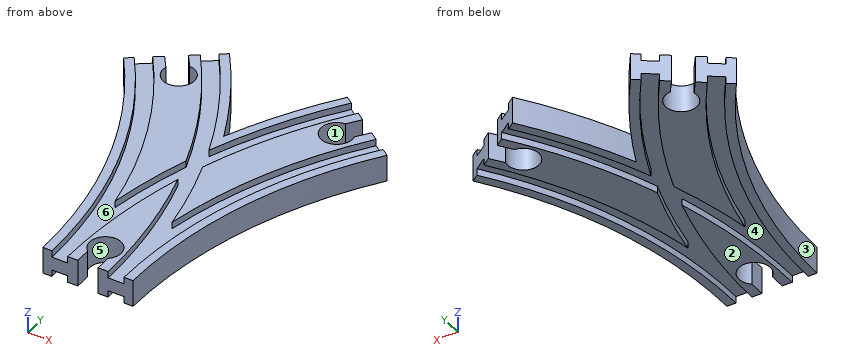
```python
from build123d import *

# Parameters (mm, degrees)
SKETCH003_W          = 7
SKETCH003_H          = 3
SKETCH004_W          = 7
SKETCH004_H          = 3
SKETCH005_W          = 7
SKETCH005_H          = 3
SKETCH006_W          = 7
SKETCH006_H          = 3
POCKET_DEPTH         = 6.001
POCKET_DEPTH_BACK    = -6.001
POCKET001_DEPTH      = 6.001
POCKET001_DEPTH_BACK = -6.001
POCKET002_DEPTH      = 6.001
POCKET002_DEPTH_BACK = -6.001


with BuildPart() as part:
    # AdditivePipe: sweep along a path in Sketch
    with BuildLine(Plane.XY) as additivepipe_path:
        ThreePointArc((0, 0), (-10.865453, 68.601773), (-42.398227, 130.488326))
    # Sketch002 → AdditivePipe (sweep)
    with BuildSketch(Plane.XZ):
        Polygon((-20, 6), (-20, -6), (-16, -6), (-16, -3), (-9, -3), (-9, -6), (9, -6), (9, -3), (16, -3), (16, -6), (20, -6), (20, 6), (16, 6), (16, 3), (9, 3), (9, 6), (-9, 6), (-9, 3), (-16, 3), (-16, 6), align=None)
    sweep(path=additivepipe_path.line)

    # AdditivePipe001: sweep along a path in Sketch001
    with BuildLine(Plane.XY) as additivepipe001_path:
        ThreePointArc((42.398227, 130.488326), (10.865453, 68.601773), (0, 0))
    # Sketch002 → AdditivePipe001 (sweep)
    with BuildSketch(Plane.XZ):
        Polygon((-20, 6), (-20, -6), (-16, -6), (-16, -3), (-9, -3), (-9, -6), (9, -6), (9, -3), (16, -3), (16, -6), (20, -6), (20, 6), (16, 6), (16, 3), (9, 3), (9, 6), (-9, 6), (-9, 3), (-16, 3), (-16, 6), align=None)
    sweep(path=additivepipe001_path.line)

    # SubtractivePipe: sweep along a path in Sketch
    with BuildLine(Plane.XY) as subtractivepipe_path:
        ThreePointArc((0, 0), (-10.865453, 68.601773), (-42.398227, 130.488326))
    # Sketch003 → SubtractivePipe (sweep, cut)
    with BuildSketch(Plane.XZ):
        with Locations((-12.5, 4.5)):
            Rectangle(SKETCH003_W, SKETCH003_H)
    sweep(path=subtractivepipe_path.line, mode=Mode.SUBTRACT)

    # SubtractivePipe001: sweep along a path in Sketch001
    with BuildLine(Plane.XY) as subtractivepipe001_path:
        ThreePointArc((42.398227, 130.488326), (10.865453, 68.601773), (0, 0))
    # Sketch003 → SubtractivePipe001 (sweep, cut)
    with BuildSketch(Plane.XZ):
        with Locations((-12.5, 4.5)):
            Rectangle(SKETCH003_W, SKETCH003_H)
    sweep(path=subtractivepipe001_path.line, mode=Mode.SUBTRACT)

    # SubtractivePipe002: sweep along a path in Sketch
    with BuildLine(Plane.XY) as subtractivepipe002_path:
        ThreePointArc((0, 0), (-10.865453, 68.601773), (-42.398227, 130.488326))
    # Sketch004 → SubtractivePipe002 (sweep, cut)
    with BuildSketch(Plane.XZ):
        with Locations((12.5, 4.5)):
            Rectangle(SKETCH004_W, SKETCH004_H)
    sweep(path=subtractivepipe002_path.line, mode=Mode.SUBTRACT)

    # SubtractivePipe003: sweep along a path in Sketch001
    with BuildLine(Plane.XY) as subtractivepipe003_path:
        ThreePointArc((42.398227, 130.488326), (10.865453, 68.601773), (0, 0))
    # Sketch004 → SubtractivePipe003 (sweep, cut)
    with BuildSketch(Plane.XZ):
        with Locations((12.5, 4.5)):
            Rectangle(SKETCH004_W, SKETCH004_H)
    sweep(path=subtractivepipe003_path.line, mode=Mode.SUBTRACT)

    # SubtractivePipe004: sweep along a path in Sketch
    with BuildLine(Plane.XY) as subtractivepipe004_path:
        ThreePointArc((0, 0), (-10.865453, 68.601773), (-42.398227, 130.488326))
    # Sketch005 → SubtractivePipe004 (sweep, cut)
    with BuildSketch(Plane.XZ):
        with Locations((-12.5, -4.5)):
            Rectangle(SKETCH005_W, SKETCH005_H)
    sweep(path=subtractivepipe004_path.line, mode=Mode.SUBTRACT)

    # SubtractivePipe005: sweep along a path in Sketch001
    with BuildLine(Plane.XY) as subtractivepipe005_path:
        ThreePointArc((42.398227, 130.488326), (10.865453, 68.601773), (0, 0))
    # Sketch005 → SubtractivePipe005 (sweep, cut)
    with BuildSketch(Plane.XZ):
        with Locations((-12.5, -4.5)):
            Rectangle(SKETCH005_W, SKETCH005_H)
    sweep(path=subtractivepipe005_path.line, mode=Mode.SUBTRACT)

    # SubtractivePipe006: sweep along a path in Sketch
    with BuildLine(Plane.XY) as subtractivepipe006_path:
        ThreePointArc((0, 0), (-10.865453, 68.601773), (-42.398227, 130.488326))
    # Sketch006 → SubtractivePipe006 (sweep, cut)
    with BuildSketch(Plane.XZ):
        with Locations((12.5, -4.5)):
            Rectangle(SKETCH006_W, SKETCH006_H)
    sweep(path=subtractivepipe006_path.line, mode=Mode.SUBTRACT)

    # SubtractivePipe007: sweep along a path in Sketch001
    with BuildLine(Plane.XY) as subtractivepipe007_path:
        ThreePointArc((42.398227, 130.488326), (10.865453, 68.601773), (0, 0))
    # Sketch006 → SubtractivePipe007 (sweep, cut)
    with BuildSketch(Plane.XZ):
        with Locations((12.5, -4.5)):
            Rectangle(SKETCH006_W, SKETCH006_H)
    sweep(path=subtractivepipe007_path.line, mode=Mode.SUBTRACT)

    # Sketch007 → Pocket (cut, two sides)
    with BuildSketch(Plane.XY) as pocket_sk:
        with BuildLine():
            Line((-4.5, 0), (4.5, 0))
            Line((4.5, 0), (4.5, 7))
            ThreePointArc((4.5, 7), (0, 19.361903), (-4.5, 7))
            Line((-4.5, 0), (-4.5, 7))
        make_face()
    extrude(amount=-POCKET_DEPTH, mode=Mode.SUBTRACT)
    extrude(pocket_sk.sketch, amount=-POCKET_DEPTH_BACK, mode=Mode.SUBTRACT)

    # Sketch008 → Pocket001 (cut, two sides)
    with BuildSketch(Plane.XY) as pocket001_sk:
        with BuildLine():
            Line((-46.038804, 127.843292), (-38.757651, 133.13336))
            Line((-38.757651, 133.13336), (-34.643154, 127.470241))
            ThreePointArc((-41.924307, 122.180173), (-31.017586, 114.824218), (-34.643154, 127.470241))
            Line((-46.038804, 127.843292), (-41.924307, 122.180173))
        make_face()
    extrude(amount=-POCKET001_DEPTH, mode=Mode.SUBTRACT)
    extrude(pocket001_sk.sketch, amount=-POCKET001_DEPTH_BACK, mode=Mode.SUBTRACT)

    # Sketch009 → Pocket002 (cut, two sides)
    with BuildSketch(Plane.XY) as pocket002_sk:
        with BuildLine():
            Line((38.757651, 133.13336), (46.038804, 127.843292))
            Line((46.038804, 127.843292), (41.924307, 122.180173))
            ThreePointArc((34.643154, 127.470241), (31.017586, 114.824218), (41.924307, 122.180173))
            Line((38.757651, 133.13336), (34.643154, 127.470241))
        make_face()
    extrude(amount=-POCKET002_DEPTH, mode=Mode.SUBTRACT)
    extrude(pocket002_sk.sketch, amount=-POCKET002_DEPTH_BACK, mode=Mode.SUBTRACT)


solid = part.part
```
The model under review builds one solid part; all positions refer to its coordinate system, in mm. Face numbers are marked on the shaded views. A direction names the side the tool comes from. Give positions to 0.01 mm unless a question says otherwise; leave off trailing zeros. Write each loop counter-clockwise with the first axis right and the second up, starting at its lowest first coordinate (ties: lowest second). Pieces come first, ordered by that corner, then holes. Notation, with made-up numbers: M 59,-33.75 L 116,-33.75 A11 cw 116,-27.75 Z; hole C 35.5,84 d7. An arc over 180 degrees is marked long. Write item = value, one per line. Start each with the question number.
Q1. We need section A-A (z = 0.5). State the section outline as (x, y) points, plus the area to 3 significant figures.
Q2. For line 1 (X direction, y = 69.5, z = -4.75); line 2 (X direction, y = 135, z = -4.5); line 3 (X direction, y = 58.5, z = 5), list the stretches that pass through material, from the lowest coordinate up.
Q3. Machinability: for the marked faces 4, 5 and 6, which of the approach directions +Z, -Z, +X, -X, +Y, -Y give a long, thin tool a straight path to every point of the face, cutting with its end or side? Answer none if there is none.
Q4. Mouldability with a two-part tool opening along X and no side actions: class the marked faces 1, 2 and 3 as released by +X, released by -X, zero draft, split by the parting line, or undercut.
Q5. We need section B-B (y = 13). State the section outline as (x, z) points, plus the area to 3 significant figures.
Q6. Clearance check with flat-ended pins moving along their axes: pin 1 (18 mm diameter, centred on x = 35.13, y = 120.49, fed in from -Z); pin 2 (2 mm diameter, centred on y = 79, z = 3.5, fed in from +X); pin 3 (6 mm diameter, centred on y = 15, z = 2, fed in from +X); pin 4 (1 mm diameter, centred on x = -38, z = -1, fed in from -Y). State where each tip first meets the part, or that it passes through.
Result set:
q1.outline = M -58.58,118.73 A202 cw -20,0 L -4.5,0 L -4.5,7 A7 cw long 4.5,7 L 4.5,0 L 20,0 A202 cw 58.58,118.73 L 46.04,127.84 L 41.92,122.18 A7 cw long 34.64,127.47 L 38.76,133.13 L 26.22,142.24 A242 ccw 0,96.33 A242 ccw -26.22,142.24 L -38.76,133.13 L -34.64,127.47 A7 cw long -41.92,122.18 L -46.04,127.84 Z
q1.area = 7,950 mm2
q2.line_1 = -32.33 to -28.08, -20.66 to -5.63, 5.63 to 20.66, 28.08 to 32.33
q2.line_2 = -36.19 to -34.55, -25.99 to -21.15, 21.15 to 25.99, 34.55 to 36.19
q2.line_3 = -28.66 to -24.48, -17.19 to -8.7, -1.47 to 1.47, 8.7 to 17.19, 24.48 to 28.66
q3.face_4 = -Z
q3.face_5 = +Z, -Z
q3.face_6 = +Z
q4.face_1 = undercut
q4.face_2 = zero draft
q4.face_3 = released by -X
q5.outline = M -20.42,-6 L -16.41,-6 L -16.41,-3 L -8.63,-3 L -8.63,-6 L -6.97,-6 L -6.97,6 L -8.63,6 L -8.63,3 L -16.41,3 L -16.41,6 L -20.42,6 Z; M 6.97,-6 L 8.63,-6 L 8.63,-3 L 16.41,-3 L 16.41,-6 L 20.42,-6 L 20.42,6 L 16.41,6 L 16.41,3 L 8.63,3 L 8.63,6 L 6.97,6 Z
q5.area = 229 mm2
q6.pin_1 = -6
q6.pin_2 = 36.52
q6.pin_3 = 20.8
q6.pin_4 = 82.24
